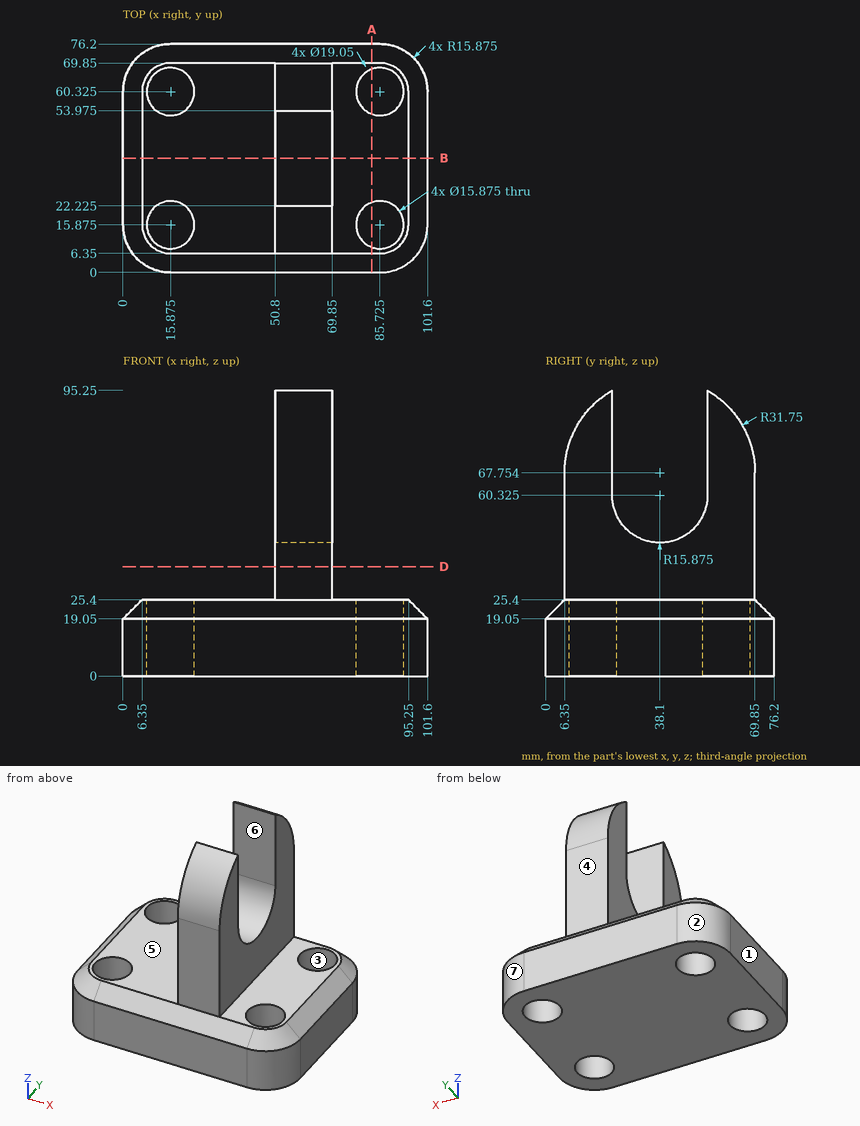
Job drawing, mm, ordinate dimensions from the low corner. One solid piece. A direction names the side the tool comes from. Round coordinates to 2 decimals unless told otherwise and drop trailing zeros. Write each loop counter-clockwise with the first axis right and the second up, starting at its lowest first coordinate (ties: lowest second). Pieces come first, ordered by that corner, then holes. Notation, with made-up numbers: M 37.25,32.5 L 70.25,32.5 A9 cw 70.25,43.5 Z; hole C 25,68.25 d9. An arc over 180 degrees is marked long. Return JSON: item names as keys, results as strings. Group by question number.
(1) Saw through at A-A on x = 83. Write the cut outline in (y, z).
(2) Saw through at D-D on z = 36.5. Write the cut outline in (x, y).
(3) Drill centre lines: probe 1 along X at (y, z) = (67.5, 18) (1 decimal); probe 2 along X at (y, z) = (13.5, 17); probe 3 along Y at (x, z) = (21.5, 8.5) (1 decimal). Where is each one in solid material? Low to high.
(4) Saw through at B-B on y = 38.1. Write the cut outline in (x, z).
(5) Pin check, flat tips, straight feed: pin 1 Ø9.5 at (x, z) = (65, 70.5) entering from -Y; pin 2 Ø20.5 at (x, y) = (15.875, 60.325) entering from +Z; pin 3 Ø15 at (x, z) = (64.5, 83) entering from +Y; pin 4 Ø14.5 at (x, y) = (85.725, 15.875) entering from -Z. Stop position of each tip, or through.
(6) Two-plate mould, pull along Y, no slides. Class the marked faces 1, 2 and 3: +Y half, -Y half, draft (parallel to the pull), parting line (faces both ways), or undercut.
(7) Which spindle directions (+Z, -Z, +X, -X, +Y, -Y) get a long thin tool onto all of the face, cutting with end or side? Do the marked faces 4, 5, 6 and 7. Say none if no direction does.
Returned:
{
 "1": {"outline": "M 0,0 L 8.42,0 L 8.42,25.4 L 6.35,25.4 L 0,19.05 Z; M 23.33,0 L 52.87,0 L 52.87,25.4 L 23.33,25.4 Z; M 67.78,0 L 76.2,0 L 76.2,19.05 L 69.85,25.4 L 67.78,25.4 Z"},
 "2": {"outline": "M 50.8,6.35 L 69.85,6.35 L 69.85,69.85 L 50.8,69.85 Z"},
 "3": {"probe 1": "1.7 to 12.5, 19.3 to 82.3, 89.1 to 99.9", "probe 2": "0.18 to 8.3, 23.45 to 78.15, 93.3 to 101.42", "probe 3": "0 to 10.3, 21.5 to 54.7, 65.9 to 76.2"},
 "4": {"outline": "M 0,0 L 101.6,0 L 101.6,19.05 L 95.25,25.4 L 69.85,25.4 L 69.85,44.45 L 50.8,44.45 L 50.8,25.4 L 6.35,25.4 L 0,19.05 Z"},
 "5": {"pin 1": "y = 6.35", "pin 2": "z = 25.4", "pin 3": "y = 68.89", "pin 4": "through"},
 "6": {"face 1": "draft", "face 2": "+Y half", "face 3": "undercut"},
 "7": {"face 4": "+Z, +X, -X, +Y", "face 5": "+Z, -X, +Y, -Y", "face 6": "+Z, +X, -X", "face 7": "+Z, -Z, +X, +Y"}
}
